Build history of the part. All positions in model axes, mm. Give positions to 0.01 mm unless a question says otherwise; leave off trailing zeros. Write each loop counter-clockwise with the first axis right and the second up, starting at its lowest first coordinate (ties: lowest second). Pieces come first, ordered by that corner, then holes. Notation, with made-up numbers: (-40, 61.5) -> (8, 61.5) arc R27 ccw to (8, 100.5) -> close; hole circle Ø6 at (-18.5, 11). An arc over 180 degrees is marked (long way). One line per question, with ' | ' between items. Start each with the question number.
(1) Drill centre lines: probe 1 along Z at (x, y) = (185, -199.9); probe 2 along Z at (x, y) = (211.5, -198.3); probe 3 along Z at (x, y) = (212, -201.8). Where is each one in solid material? Low to high. Write a range as from..to.
(2) Band-saw the part on A-A, the plane x = 185. Give the cut face in (y, z).
(3) Pull direction Z, two halves, no side cores. Call faces 1 (the flat face through (185, -198, 15)), 2 (the cylindrical face through (213.615, -199.972, -0.511)), 3 (the cylindrical face through (199.802, -199.972, 12.903)): released by +Z, released by -Z, zero draft, split by the parting line, or undercut.
(4) Pin check, flat tip, straight feed: P1, Ø1.5, axis at x = 199.5, y = -199.5, coming from the -Z side. Stop position of the tip, or through.
(5) Band-saw the part on D-D, the plane z = 13. Give the cut face in (x, y), and give its area (3 significant figures).
(6) Band-saw the part on C-C, the plane x = 209.5. Give the cut face in (y, z), and give its area (3 significant figures).
(7) Band-saw the part on B-B, the plane y = -199.3. Give the cut face in (x, z), and give its area (3 significant figures).
from build123d import *

# Parameters (mm, degrees)
CYLINDER052_R          = 2.8
CYLINDER052_DEPTH      = 10
CYLINDER052_ROLL_ANGLE = -90
CYLINDER047_R          = 2.2
CYLINDER047_DEPTH      = 26
CYLINDER047_ROLL_ANGLE = -90
ARRAY018_X_COUNT       = 2
ARRAY018_X_PITCH       = 8
ARRAY018_Z_COUNT       = 2
ARRAY018_Z_PITCH       = 9
CYLINDER045_R          = 30
CYLINDER045_DEPTH      = 4
CYLINDER045_ROLL_ANGLE = -90


with BuildPart() as obj1:
    # Cylinder052 → Cylinder052 (new body)
    with BuildSketch(Plane.XY):
        Circle(CYLINDER052_R)
    extrude(amount=CYLINDER052_DEPTH)


with BuildPart() as obj1_1:
    # Cylinder052 roll: moved
    add(obj1.part.rotate(Axis((0, 0, 0), (1, 0, 0)), CYLINDER052_ROLL_ANGLE))


with BuildPart() as obj1_2:
    # Cylinder052 placement: moved
    add(obj1_1.part.moved(Location((185, 18, 8.5))))


with BuildPart() as obj2:
    # Cylinder047 → Cylinder047 (new body)
    with BuildSketch(Plane.XY):
        Circle(CYLINDER047_R)
    extrude(amount=CYLINDER047_DEPTH)


with BuildPart() as obj2_1:
    # Cylinder047 roll: moved
    add(obj2.part.rotate(Axis((0, 0, 0), (1, 0, 0)), CYLINDER047_ROLL_ANGLE))


with BuildPart() as obj2_2:
    # Cylinder047 placement: moved
    add(obj2_1.part.moved(Location((202, 0, 4))))

    # Array018 X: obj2_2


with BuildPart() as obj2_3:
    add(obj2_2.part)
    with Locations(*[(i * ARRAY018_X_PITCH, 0, 0) for i in range(1, ARRAY018_X_COUNT)]):
        add(obj2_2.part)

    # Array018 Z: obj2_2


with BuildPart() as obj2_4:
    add(obj2_3.part)
    with Locations(*[(0, 0, i * ARRAY018_Z_PITCH) for i in range(1, ARRAY018_Z_COUNT)]):
        add(obj2_3.part)


with BuildPart() as obj3:
    # Cylinder045 → Cylinder045 (new body)
    with BuildSketch(Plane.XY):
        Circle(CYLINDER045_R)
    extrude(amount=CYLINDER045_DEPTH)


with BuildPart() as obj3_1:
    # Cylinder045 roll: moved
    add(obj3.part.rotate(Axis((0, 0, 0), (1, 0, 0)), CYLINDER045_ROLL_ANGLE))


with BuildPart() as obj3_2:
    # Cylinder045 placement: moved
    add(obj3_1.part.moved(Location((185, 20, 8.5))))

    # Cut053: cut obj2
    add(obj2_4.part, mode=Mode.SUBTRACT)

    # Cut056: cut obj1
    add(obj1_2.part, mode=Mode.SUBTRACT)


with BuildPart() as obj4:
    # Part__Mirroring020: instance of obj3
    add(obj3_2.part.mirror(Plane(origin=(0, 0, 0), x_dir=(1, 0, 0), z_dir=(0, 1, 0))))


with BuildPart() as obj4_1:
    # Part__Mirroring020 placement: moved
    add(obj4.part.moved(Location((0, -178, 0))))


solid = obj4_1.part
Results:
1) probe 1: z = -21.5..5.7, 11.3..38.5 | probe 2: z = -5.56..2.39, 5.61..11.39, 14.61..22.56 | probe 3: z = -4.58..3.08, 4.92..12.08, 13.92..21.58
2) outline: (-202, -21.5) -> (-198, -21.5) -> (-198, 5.7) -> (-202, 5.7) -> close; (-202, 11.3) -> (-198, 11.3) -> (-198, 38.5) -> (-202, 38.5) -> close
3) face 1: zero draft | face 2: split by the parting line | face 3: undercut
4) P1: stops at z = -18.16
5) outline: (155.34, -202) -> (199.8, -202) -> (199.8, -198) -> (155.34, -198) -> close; (204.2, -202) -> (207.8, -202) -> (207.8, -198) -> (204.2, -198) -> close; (212.2, -202) -> (214.66, -202) -> (214.66, -198) -> (212.2, -198) -> close | area: 202 mm²
6) outline: (-202, -8.81) -> (-198, -8.81) -> (-198, 1.86) -> (-202, 1.86) -> close; (-202, 6.14) -> (-198, 6.14) -> (-198, 10.86) -> (-202, 10.86) -> close; (-202, 15.14) -> (-198, 15.14) -> (-198, 25.81) -> (-202, 25.81) -> close | area: 104 mm²
7) outline: circle Ø60 at (185, 8.5); hole circle Ø5.6 at (185, 8.5); hole circle Ø4.4 at (202, 4); hole circle Ø4.4 at (202, 13); hole circle Ø4.4 at (210, 4); hole circle Ø4.4 at (210, 13) | area: 2,740 mm²
